Can you work these out from the drawing? Everything is in mm from the part's minimum corner. A direction names the side the tool comes from. Coordinates: 2 decimals unless noted, no trailing zeros. Order: outer loops, then holes, each group sorted by start corner. A loop starts at its lowest first (then second) coordinate and runs counter-clockwise, first axis right, second up. Notation, with made-up numbers: (30, 42.25) -> (73, 42.25) arc R11 cw to (73, 50.25) -> close; hole circle Ø10 at (47, 28.5). An arc over 180 degrees is marked (long way). Answer in a Markdown table with one row per item.
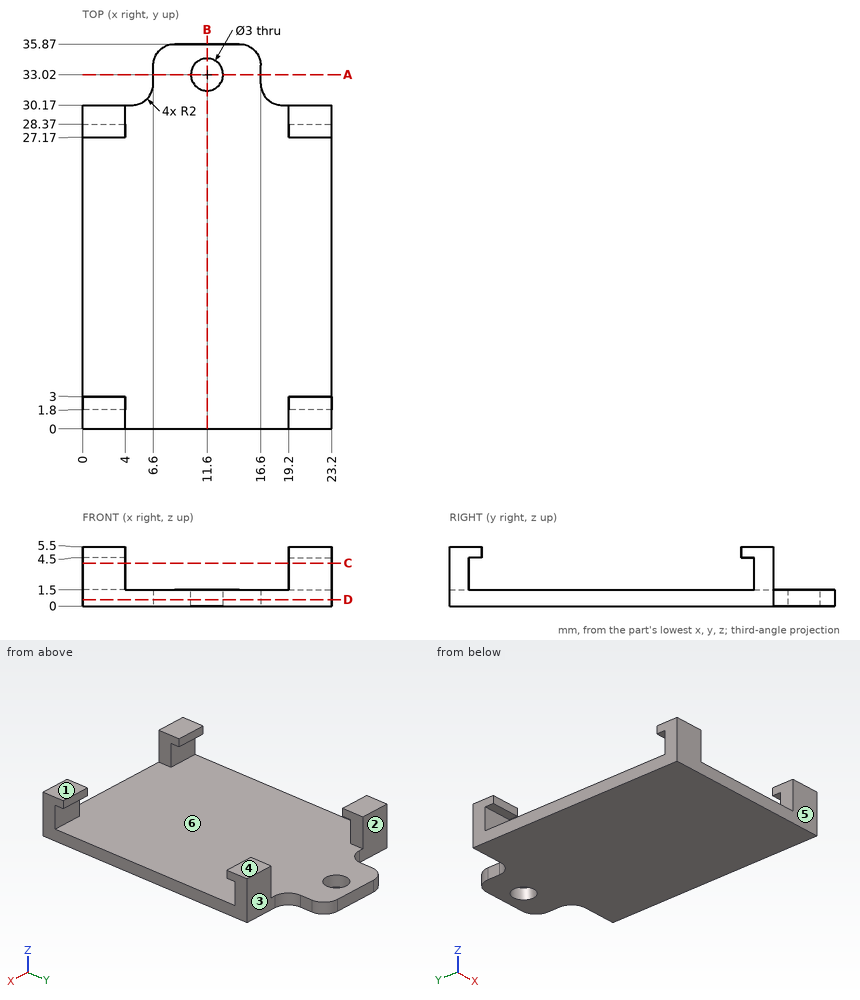
(1) Suppose I cut it at D-D (z = 0.6). Please give me the cut outline in (x, y), and give its area (3 significant figures).
Response values:
| item | result |
|---|---|
| outline | (0, 0) -> (23.2, 0) -> (23.2, 30.17) -> (18.6, 30.17) arc R2 cw to (16.6, 32.17) -> (16.6, 33.87) arc R2 ccw to (14.6, 35.87) -> (8.6, 35.87) arc R2 ccw to (6.6, 33.87) -> (6.6, 32.17) arc R2 cw to (4.6, 30.17) -> (0, 30.17) -> close; hole circle Ø3 at (11.6, 33.02) |
| area | 750 mm2 |
(2) Suppose I cut it at B-B (x = 11.6). Please give me the cut outline in (y, z).
Response values:
| item | result |
|---|---|
| outline | (0, 0) -> (31.52, 0) -> (31.52, 1.5) -> (0, 1.5) -> close; (34.52, 0) -> (35.87, 0) -> (35.87, 1.5) -> (34.52, 1.5) -> close |
(3) Suppose I cut it at A-A (y = 33.02). Please give me the cut outline in (x, z), and give its area (3 significant figures).
Response values:
| item | result |
|---|---|
| outline | (6.6, 0) -> (10.1, 0) -> (10.1, 1.5) -> (6.6, 1.5) -> close; (13.1, 0) -> (16.6, 0) -> (16.6, 1.5) -> (13.1, 1.5) -> close |
| area | 10.5 mm2 |
(4) Suppose I cut it at C-C (z = 4). Please give me the cut outline in (x, y).
Response values:
| item | result |
|---|---|
| outline | (0, 0) -> (4, 0) -> (4, 1.8) -> (0, 1.8) -> close; (0, 28.37) -> (4, 28.37) -> (4, 30.17) -> (0, 30.17) -> close; (19.2, 0) -> (23.2, 0) -> (23.2, 1.8) -> (19.2, 1.8) -> close; (19.2, 28.37) -> (23.2, 28.37) -> (23.2, 30.17) -> (19.2, 30.17) -> close |
(5) On a 3-axis mill with a long thin cutter (end or side, diameter ignored), from which of +Z, -Z, +X, -X, +Y, -Y can I reach the whole of each face in a straight line? I mean the marked faces 1, 2 and 3. Say none if no direction works.
Response values:
| item | result |
|---|---|
| face 1 | +Z, +X, -X, +Y, -Y |
| face 2 | +Z, -Z, -X, +Y |
| face 3 | +Z, -Z, +X, +Y |
(6) I need wall thicknesses on line 1 (X direction, y = 33.02, z = 0.7); line 2 (Z direction, x = 9.5, y = 30); line 3 (Y direction, x = 18.5, z = 1.3). Which ranges of each line are inside material? Lowest first, please. Write a range as [from, to].
Response values:
| item | result |
|---|---|
| line 1 | [6.6, 10.1], [13.1, 16.6] |
| line 2 | [0, 1.5] |
| line 3 | [0, 30.17] |
(7) We'd pull the mould along Y, two halves only. Please class the marked faces 4, 5 and 6: +Y half, -Y half, draft (parallel to the pull), parting line (faces both ways), or undercut.
Response values:
| item | result |
|---|---|
| face 4 | draft |
| face 5 | -Y half |
| face 6 | undercut |
(8) Will these pins go through, and if not, where does the flat tip stop? pin 1 Ø2 at (x, y) = (15.5, 27.5) entering from +Z; pin 2 Ø0.5 at (x, z) = (21.5, 5) entering from +Y; pin 3 Ø1.2 at (y, z) = (33, 0.5) entering from -X.
Response values:
| item | result |
|---|---|
| pin 1 | z = 1.5 |
| pin 2 | y = 30.17 |
| pin 3 | x = 6.6 |
